CAD build for the part. Positions are in the model's coordinates, mm. Face numbers are marked on the shaded views. A direction names the side the tool comes from. Coordinates: 2 decimals unless noted, no trailing zeros. Loops run counter-clockwise (first coordinate to the right, second up) from the corner with the lowest first, then second, coordinate; pieces in that order, holes last. Notation, with made-up numbers: (-3, -9.5) -> (43, -9.5) arc R19 cw to (43, 23.5) -> close; hole circle Ø2 at (61, 58). An arc over 180 degrees is marked (long way). Return JSON: item names as keys, results as strings. Group by question number.
(1) Saw through at B-B on z = -20. Write the cut outline in (x, y).
(2) Probe L1, parallel to Z at x = 20, y = 3.6; L2, parallel to X at y = 9, z = -30.5; L3, parallel to Y at x = 54, z = -12.5. List the from-to ranges inside material, lowest first.
(3) Saw through at A-A on x = 68. Write the cut outline in (y, z), then the cut area to 3 significant figures.
(4) Tool access for the marked faces 1, 2 and 3: list every direction of +Z, -Z, +X, -X, +Y, -Y with a clear straight run to the whole face (end or side of a thin tool).
(5) Flat gauge pins, fed straight in: pin 1 Ø10 at (y, z) = (35.5, -32.5) entering from -X; pin 2 Ø1 at (x, z) = (59.5, -34) entering from -Y; pin 3 Ø5 at (y, z) = (11.5, -14) entering from +X. Where does each tip first touch, or does it go through?
(6) Saw through at D-D on x = 15. Write the cut outline in (y, z).
(7) Saw through at C-C on z = -31. Write the cut outline in (x, y).
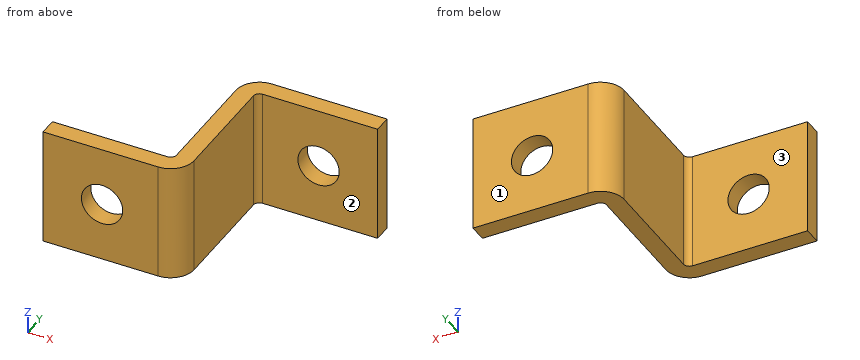
```python
from build123d import *

# Parameters (mm, degrees)
SKETCH1_W                      = 88
SKETCH1_H                      = 54
BOSS_EXTRUDE1_DEPTH            = 40
SKETCH2_W                      = 41
SKETCH2_H                      = 48
CUT_EXTRUDE1_DEPTH             = 41
SKETCH3_W                      = 41
SKETCH3_H                      = 48
CUT_EXTRUDE2_DEPTH             = 41
F_14_0_14_DIAMETER_HOLE1_D     = 14
F_14_0_14_DIAMETER_HOLE1_DEPTH = 54
F_14_0_14_DIAMETER_HOLE2_D     = 14
F_14_0_14_DIAMETER_HOLE2_DEPTH = 54
FILLET1_R                      = 2
FILLET2_R                      = 8


with BuildPart() as part:
    # Sketch1 → Boss-Extrude1 (new body)
    with BuildSketch(Plane(origin=(0, 0, -40), x_dir=(-1, 0, 0), z_dir=(0, 0, -1))):
        with Locations((-44, 27)):
            Rectangle(SKETCH1_W, SKETCH1_H)
    extrude(amount=-BOSS_EXTRUDE1_DEPTH)

    # Sketch2 → Cut-Extrude1 (cut, through all)
    with BuildSketch(Plane.XY):
        with Locations((20.5, 30)):
            Rectangle(SKETCH2_W, SKETCH2_H)
    extrude(amount=-CUT_EXTRUDE1_DEPTH, mode=Mode.SUBTRACT)

    # Sketch3 → Cut-Extrude2 (cut, through all)
    with BuildSketch(Plane.XY):
        with Locations((67.5, 24)):
            Rectangle(SKETCH3_W, SKETCH3_H)
    extrude(amount=-CUT_EXTRUDE2_DEPTH, mode=Mode.SUBTRACT)

    # Ø14.0 (14) Diameter Hole1
    with Locations(Plane(origin=(0, 0, 0), x_dir=(-1, 0, 0), z_dir=(0, -1, 0))):
        with Locations((-20, 20)):
            Hole(F_14_0_14_DIAMETER_HOLE1_D / 2, depth=F_14_0_14_DIAMETER_HOLE1_DEPTH)

    # Ø14.0 (14) Diameter Hole2
    with Locations(Plane(origin=(0, 54, 0), x_dir=(1, 0, 0), z_dir=(0, 1, 0))):
        with Locations((68, 20)):
            Hole(F_14_0_14_DIAMETER_HOLE2_D / 2, depth=F_14_0_14_DIAMETER_HOLE2_DEPTH)

    # Fillet1
    fillet1_edges = [part.edges().sort_by_distance(p)[0] for p in [
        (41, 6, -20),
        (47, 48, -20),
    ]]
    fillet(fillet1_edges, radius=FILLET1_R)

    # Fillet2
    fillet2_edges = [part.edges().sort_by_distance(p)[0] for p in [
        (41, 54, -20),
        (47, 0, -20),
    ]]
    fillet(fillet2_edges, radius=FILLET2_R)


solid = part.part
```
Geometry results:
{
 "1": {"outline": "(0, 0) -> (13, 0) -> (13, 6) -> (0, 6) -> close; (27, 0) -> (39, 0) arc R8 ccw to (47, 8) -> (47, 46) arc R2 cw to (49, 48) -> (61, 48) -> (61, 54) -> (49, 54) arc R8 ccw to (41, 46) -> (41, 8) arc R2 cw to (39, 6) -> (27, 6) -> close; (75, 48) -> (88, 48) -> (88, 54) -> (75, 54) -> close"},
 "2": {"L1": "-40 to -27, -13 to 0", "L2": "41 to 47", "L3": "48 to 54"},
 "3": {"outline": "(48, -40) -> (54, -40) -> (54, -27) -> (48, -27) -> close; (48, -13) -> (54, -13) -> (54, 0) -> (48, 0) -> close", "area": "156 mm²"},
 "4": {"face 1": "+Z, -Z, +X, -X, +Y", "face 2": "+Z, -Z, +X, -Y", "face 3": "+Z, -Z, -X, +Y"},
 "5": {"pin 1": "x = 41", "pin 2": "y = 48", "pin 3": "x = 47"},
 "6": {"outline": "(0, -40) -> (6, -40) -> (6, -24.9) -> (0, -24.9) -> close; (0, -15.1) -> (6, -15.1) -> (6, 0) -> (0, 0) -> close"},
 "7": {"outline": "(0, 0) -> (39, 0) arc R8 ccw to (47, 8) -> (47, 46) arc R2 cw to (49, 48) -> (88, 48) -> (88, 54) -> (49, 54) arc R8 ccw to (41, 46) -> (41, 8) arc R2 cw to (39, 6) -> (0, 6) -> close"}
}
